For this review, take the finished solid that the model builds, in its own axes (mm). A direction names the side the tool comes from. Round coordinates to 2 decimals unless told otherwise and drop trailing zeros. Order: outer loops, then holes, each group sorted by start corner. A loop starts at its lowest first (then second) coordinate and runs counter-clockwise, first axis right, second up. Notation, with made-up numbers: M -19.75,-10.75 L 39.25,-10.75 A24 ccw 39.25,22.25 Z; hole C -18.75,74.25 d11. An arc over 180 degrees is marked long. Put each result on its own line as item: value.
from build123d import *

# Parameters (mm, degrees)
ESQUISSE1_R        = 1.5
ESQUISSE1_R_2      = 2.5
BOSS_EXTRU_1_DEPTH = 2
BOSS_EXTRU_2_DEPTH = 50
CONG_1_R           = 0.5
ESQUISSE3_W        = 8
ESQUISSE3_H        = 8
ESQUISSE3_R        = 1.6
BOSS_EXTRU_4_DEPTH = 8


with BuildPart() as part:
    # Esquisse1 → Boss.-Extru.1 (new body)
    with BuildSketch(Plane.XY):
        with BuildLine():
            Line((-7.341000528, 15), (-15, 7.5))
            Line((-15, 7.5), (-15, 0))
            Line((-15, 0), (-13, 0))
            ThreePointArc((-13, 0), (0, -13), (13, 0))
            Line((13, 0), (15, 0))
            Line((15, 0), (15, 7.5))
            Line((15, 7.5), (7.658999472, 15))
            Line((7.658999472, 15), (-7.341000528, 15))
        make_face()
        with Locations((0, 10)):
            Circle(ESQUISSE1_R, mode=Mode.SUBTRACT)
        with Locations((-10, 0)):
            Circle(ESQUISSE1_R, mode=Mode.SUBTRACT)
        with Locations((0, -10)):
            Circle(ESQUISSE1_R, mode=Mode.SUBTRACT)
        Circle(ESQUISSE1_R_2, mode=Mode.SUBTRACT)
        with Locations((10, 0)):
            Circle(ESQUISSE1_R, mode=Mode.SUBTRACT)
    extrude(amount=BOSS_EXTRU_1_DEPTH)

    # Esquisse2 → Boss.-Extru.2 (add)
    with BuildSketch(Plane(origin=(0, 0, 0), x_dir=(-1, 0, 0), z_dir=(0, 0, -1))):
        with BuildLine():
            ThreePointArc((13, 0), (9.192388155, -9.192388155), (0, -13))
            Line((0, -13), (0, -15))
            ThreePointArc((0, -15), (10.606601718, -10.606601718), (15, 0))
            Line((15, 0), (13, 0))
        make_face()
        with BuildLine():
            Line((0, -15), (0, -13))
            ThreePointArc((0, -13), (-9.192388155, -9.192388155), (-13, 0))
            Line((-13, 0), (-15, 0))
            ThreePointArc((-15, 0), (-10.606601718, -10.606601718), (0, -15))
        make_face()
        with BuildLine():
            Line((0, -20), (0, -15))
            ThreePointArc((0, -15), (-10.606601718, -10.606601718), (-15, 0))
            Line((-15, 0), (-15, -20))
            Line((-15, -20), (0, -20))
        make_face()
        with BuildLine():
            ThreePointArc((15, 0), (10.606601718, -10.606601718), (0, -15))
            Line((0, -15), (0, -20))
            Line((0, -20), (15, -20))
            Line((15, -20), (15, 0))
        make_face()
    extrude(amount=-BOSS_EXTRU_2_DEPTH)

    # Congé1
    cong_1_edges = [part.edges().sort_by_distance(p)[0] for p in [
        (-2.5, 0, 0),
    ]]
    fillet(cong_1_edges, radius=CONG_1_R)

    # Esquisse3 → Boss.-Extru.4 (add)
    # profile 1 of 4: a face of its own
    with BuildSketch(Plane.XZ.offset(20)):
        with Locations((19, 12)):
            Rectangle(ESQUISSE3_W, ESQUISSE3_H)
        with Locations(Location((19, 12, 0), (0, 0, 270))):
            Circle(ESQUISSE3_R, mode=Mode.SUBTRACT)
    # profile 2 of 4: a face of its own
    with BuildSketch(Plane.XZ.offset(20)):
        with Locations((19, 4)):
            Rectangle(ESQUISSE3_W, ESQUISSE3_H)
        with Locations(Location((19, 4, 0), (0, 0, 270))):
            Circle(ESQUISSE3_R, mode=Mode.SUBTRACT)
    # profile 3 of 4: a face of its own
    with BuildSketch(Plane.XZ.offset(20)):
        with Locations((11, 54)):
            Rectangle(ESQUISSE3_W, ESQUISSE3_H)
        with Locations(Location((11, 54, 0), (0, 0, 270))):
            Circle(ESQUISSE3_R, mode=Mode.SUBTRACT)
    # profile 4 of 4: a face of its own
    with BuildSketch(Plane.XZ.offset(20)):
        with Locations((-11, 54)):
            Rectangle(ESQUISSE3_W, ESQUISSE3_H)
        with Locations(Location((-11, 54, 0), (0, 0, 270))):
            Circle(ESQUISSE3_R, mode=Mode.SUBTRACT)
    extrude(amount=-BOSS_EXTRU_4_DEPTH)


solid = part.part
(1) Add section D-D on y = -10. Give the boundary of the cut face in (x, z).
A:
outline: M -15,0 L -1.5,0 L -1.5,2 L -8.31,2 L -8.31,50 L -15,50 Z; M 1.5,0 L 15,0 L 15,50 L 8.31,50 L 8.31,2 L 1.5,2 Z
(2) Add section B-B on x = 19. Give the boundary of the cut face in (y, z), then the cut area to 3 significant figures.
A:
outline: M -20,0 L -12,0 L -12,2.4 L -20,2.4 Z; M -20,5.6 L -12,5.6 L -12,10.4 L -20,10.4 Z; M -20,13.6 L -12,13.6 L -12,16 L -20,16 Z
area: 76.8 mm2
(3) Add section A-A on z = 12. Give the boundary of the cut face in (x, y).
A:
outline: M -15,-20 L 17.4,-20 L 17.4,-12 L 15,-12 L 15,0 L 13,0 A13 cw -13,0 L -15,0 Z; M 20.6,-20 L 23,-20 L 23,-12 L 20.6,-12 Z
(4) To check wall thickness, follow L1, parallel to X at y = -17, z = 54; L2, parallel to X at y = -18, z = 4; L3, parallel to Y at x = -8, z = 53. State the ranges of each line that lie inside material, in increasing order.
A:
L1: x = -15 to -12.6, -9.4 to -7, 7 to 9.4, 12.6 to 15
L2: x = -15 to 17.4, 20.6 to 23
L3: y = -20 to -12
(5) For faces 4 (the face through (-0.325, -11.464, 0.986)), 5 (the face through (19, -12, 8)), 6 (the face through (7, -16, 54)), 7 (the face through (0, 4, 2)), 8 (the face through (-11, -12, 56)), list the 3-axis set-ups (+Z, -Z, +X, -X, +Y, -Y) from which the entire face can be reached by the end or side of a thin tool; tool diameter is ignored.
A:
face 4: +Z, -Z
face 5: +Z, -Z, +X, +Y
face 6: +Z, +Y, -Y
face 7: +Z, +Y
face 8: +Z, +X, -X, +Y
(6) Insertion check: pin 1 Ø10 at (x, z) = (19, 42) entering from +Y; pin 2 Ø2 at (y, z) = (-12.5, 23.5) entering from +X; pin 3 Ø6.5 at (x, z) = (12.5, 55) entering from +Y. Each pin has a flat end and moves straight along its axis. Give the tip position at first contact, or say it passes through.
A:
pin 1: stops at y = 0
pin 2: stops at x = 15
pin 3: stops at y = -12
(7) Add section C-C on z = 54. Give the boundary of the cut face in (x, y), then the cut area to 3 significant figures.
A:
outline: M -15,-20 L -12.6,-20 L -12.6,-12 L -15,-12 Z; M -9.4,-20 L -7,-20 L -7,-12 L -9.4,-12 Z; M 7,-20 L 9.4,-20 L 9.4,-12 L 7,-12 Z; M 12.6,-20 L 15,-20 L 15,-12 L 12.6,-12 Z
area: 76.8 mm2
(8) Draft analysis for pull direction Y (two halves, no side actions). For faces 1 (the face through (-11.12, 11.3, 0.99)), 2 (the face through (-0.325, 8.536, 0.986)), 3 (the face through (0, -14, 50)), state which applies: released by +Y, released by -Y, zero draft, split by the parting line, or undercut.
A:
face 1: released by +Y
face 2: undercut
face 3: zero draft
